The model under review builds one solid part; all positions refer to its coordinate system, in mm. A direction names the side the tool comes from. Coordinates: 2 decimals unless noted, no trailing zeros. Write each question's results on one line, items separated by ' | '.
```python
from build123d import *

# Parameters (mm, degrees)
F1_DEPTH    = 6.35
F0_W        = 6.35
F0_H        = 177.8
F2_DEPTH    = 3.81
F3_R        = 1.5875
F4_DEPTH    = 177.8
F5_R        = 1.5875
F6_DEPTH    = 6.35
F7_R        = 5.08
F8_T1_DEPTH = 232.7005208253
F8_T3_DEPTH = 188.2505208253


# Not quite as in the source:
# - a fillet or chamfer that OpenCascade refuses, or shapes differently, is made with other operations: its cross-section is extruded or revolved along the edge and cut away or added


with BuildPart() as f1:
    # F0 (on Top) → F1 (new body)
    with BuildSketch(Plane.XY):
        Polygon((-11.6160511255, 102.6400476694), (-11.6160511255, -75.1599523306), (-11.6160511255, -94.2099523306), (159.8339488745, -94.2099523306), (159.8339488745, 121.6900476694), (-11.6160511255, 121.6900476694), align=None)
    extrude(amount=-F1_DEPTH)

    # F0 (on Top) → F2 (join)
    with BuildSketch(Plane.XY):
        with Locations((-14.7910511255, 13.7400476694)):
            Rectangle(F0_W, F0_H)
    extrude(amount=-F2_DEPTH)

    # F3 (on face) → F4 (cut)
    with BuildSketch(Plane.XZ.offset(75.1599523306)):
        with Locations((-14.7910511255, -1.905)):
            Circle(F3_R)
    extrude(amount=-F4_DEPTH, mode=Mode.SUBTRACT)

    # F5 (on face) → F6 (cut)
    with BuildSketch(Plane.XY):
        with Locations((13.7839488745, 13.7400476694)):
            Circle(F5_R)
    extrude(amount=-F6_DEPTH, mode=Mode.SUBTRACT)

    # F7
    f7_edges = [f1.edges().sort_by_distance(p)[0] for p in [
        (74.108949, -94.209952, 0),
        (159.833949, 13.740048, 0),
        (74.108949, 121.690048, 0),
    ]]
    fillet(f7_edges, radius=F7_R)

    # F8: fillet of radius 5.08 on 3 edges, made by hand

    # F8_s2 → F8_t1 (cut)
    with BuildSketch(Plane.XZ.offset(-130.090308082)):
        with BuildLine():
            ThreePointArc((156.4738447094, -6.35), (158.2698959336, -6.0219048812), (159.8339488745, -5.08))
            Line((159.8339488745, -5.08), (159.8339488745, -6.35))
            Line((159.8339488745, -6.35), (156.4738447094, -6.35))
        make_face()
    extrude(amount=F8_T1_DEPTH, mode=Mode.SUBTRACT)

    # F8_s4 → F8_t3 (cut)
    with BuildSketch(Plane.YZ.offset(-20.0163115382)):
        with BuildLine():
            ThreePointArc((-90.8498481655, -6.35), (-92.6458993898, -6.0219048812), (-94.2099523306, -5.08))
            Line((-94.2099523306, -5.08), (-94.2099523306, -6.35))
            Line((-94.2099523306, -6.35), (-90.8498481655, -6.35))
        make_face()
        with BuildLine():
            ThreePointArc((121.6900476694, -5.08), (120.1259947286, -6.0219048812), (118.3299435044, -6.35))
            Line((118.3299435044, -6.35), (121.6900476694, -6.35))
            Line((121.6900476694, -6.35), (121.6900476694, -5.08))
        make_face()
    extrude(amount=F8_T3_DEPTH, mode=Mode.SUBTRACT)


solid = f1.part
```
Q1. Machinability: for faces 1 (the flat face through (-15, 15, -3.81)), 2 (the cylindrical face through (72.909, 120.162, -1.449)), which of the approach directions +Z, -Z, +X, -X, +Y, -Y give a long, thin tool a straight path to every point of the face, cutting with its end or side? Answer none if there is none.
Solution:
face 1: -Z, -X, +Y, -Y | face 2: +Z, +X, -X, +Y
Q2. For line 1 (X direction, y = -20.5, z = -4.5); line 2 (X direction, y = -52.5, z = -1.75); line 3 (X direction, y = 72, z = -0.75), list the stretches that pass through material, from the lowest coordinate up. Write a range as from..to.
Solution:
line 1: -11.62..159.8 | line 2: -17.97..-16.37, -13.21..158.59 | line 3: -17.97..-15.88, -13.7..157.41
Q3. Clearance check with flat-ended pins moving along their axes: P1, Ø3, axis at x = -13.5, z = -2.5, coming from the +Y side; P2, Ø1.9, axis at x = -14.79, z = -1.9, coming from the -Y side. State where each tip first meets the part, or that it passes through.
Solution:
P1: y = 102.64 | P2: through
